```python
from build123d import *

# Parameters (mm, degrees)
SKETCH1_R           = 4
SKETCH1_R_2         = 1.7
SKETCH1_R_3         = 11
BOSS_EXTRUDE1_DEPTH = 3
FILLET1_R           = 10
SKETCH2_R           = 1.25
SKETCH2_R_2         = 1.255555556
CUT_EXTRUDE1_DEPTH  = 3


with BuildPart() as part:
    # Sketch1 → Boss-Extrude1 (new body)
    with BuildSketch(Plane(origin=(0, 0, 0), x_dir=(1, 0, 0), z_dir=(0, 1, 0))):
        Polygon((20, -64), (-20, -64), (-60, -7), (-60, 21.5), (-45.5, 50), (-31, 50), (-31, 19), (31, 19), (31, 50), (45.5, 50), (60, 21.5), (60, -7), align=None)
        with Locations((0, -10)):
            Circle(SKETCH1_R, mode=Mode.SUBTRACT)
        with Locations((-40, 0)):
            Circle(SKETCH1_R, mode=Mode.SUBTRACT)
        with Locations((40, 0)):
            Circle(SKETCH1_R, mode=Mode.SUBTRACT)
        with Locations((-15.5, -23.5)):
            Circle(SKETCH1_R_2, mode=Mode.SUBTRACT)
        with Locations((15.5, -23.5)):
            Circle(SKETCH1_R_2, mode=Mode.SUBTRACT)
        with Locations((15.5, -54.5)):
            Circle(SKETCH1_R_2, mode=Mode.SUBTRACT)
        with Locations((-15.5, -54.5)):
            Circle(SKETCH1_R_2, mode=Mode.SUBTRACT)
        with Locations((0, -39)):
            Circle(SKETCH1_R_3, mode=Mode.SUBTRACT)
    extrude(amount=BOSS_EXTRUDE1_DEPTH)

    # Fillet1
    fillet1_edges = [part.edges().sort_by_distance(p)[0] for p in [
        (45.5, 1.5, -50),
        (60, 1.5, -21.5),
        (60, 1.5, 7),
        (20, 1.5, 64),
        (-20, 1.5, 64),
        (-60, 1.5, 7),
        (-60, 1.5, -21.5),
        (-45.5, 1.5, -50),
    ]]
    fillet(fillet1_edges, radius=FILLET1_R)

    # Sketch2 → Cut-Extrude1 (cut)
    with BuildSketch(Plane(origin=(0, 3, 0), x_dir=(1, 0, 0), z_dir=(0, 1, 0))):
        with Locations((-32.400459523, -28.920654821)):
            Circle(SKETCH2_R)
        with Locations((32.400459523, -28.920654821)):
            Circle(SKETCH2_R)
        with Locations((0, 9)):
            Circle(SKETCH2_R)
        with Locations((-41, 36.792031786)):
            Circle(SKETCH2_R)
        with Locations((41, 36.792031786)):
            Circle(SKETCH2_R_2)
    extrude(amount=-CUT_EXTRUDE1_DEPTH, mode=Mode.SUBTRACT)


solid = part.part
```
Build history of the part. All positions in model axes, mm. A direction names the side the tool comes from. Round coordinates to 2 decimals unless told otherwise and drop trailing zeros. Write each loop counter-clockwise with the first axis right and the second up, starting at its lowest first coordinate (ties: lowest second). Pieces come first, ordered by that corner, then holes. Notation, with made-up numbers: (20.25, -7.75) - (41.25, -7.75) arc R21 cw to (41.25, 29.25) - close; hole circle Ø11 at (85, 56). An arc over 180 degrees is marked (long way). Answer as CSV lines item,"result".
Q1. Pull direction Z, two halves, no side cores. Call faces 3 (the cylindrical face through (-31.246, 1.521, 29.399)), 4 (the cylindrical face through (-19.354, 1.521, 62.903)), 5 (the cylindrical face through (17.07, 1.48, 55.15)), 6 (the flat face through (-35, 1, -50)): +Z half, -Z half, draft (parallel to the pull), parting line (faces both ways), or undercut.
Report:
face 3,"undercut"
face 4,"+Z half"
face 5,"undercut"
face 6,"-Z half"
Q2. Drill centre lines: probe 1 along Z at (x, y) = (0, 1.5); probe 2 along X at (y, z) = (2.45, 0); probe 3 along Z at (x, y) = (15.5, 1.25). Where is each one in solid material? Low to high. Write a range as [from, to].
Report:
probe 1,"z = [-19, -10.25], [-7.75, 6], [14, 28], [50, 64]"
probe 2,"x = [-60, -44], [-36, 36], [44, 60]"
probe 3,"z = [-19, 21.8], [25.2, 52.8], [56.2, 63.98]"
Q3. Tool access for faces 1 (the cylindrical face through (-43.2, 1.5, 2.4)), 2 (the flat face through (-31, 1, -35)): list every direction of +Z, -Z, +X, -X, +Y, -Y with a clear straight run to the whole face (end or side of a thin tool).
Report:
face 1,"+Y, -Y"
face 2,"-Z, +Y, -Y"
Q4. Cut at C-C (z = 54.5). Write the cut outline in (x, y).
Report:
outline,"(-26.67, 0) - (-17.2, 0) - (-17.2, 3) - (-26.67, 3) - close; (-13.8, 0) - (13.8, 0) - (13.8, 3) - (-13.8, 3) - close; (17.2, 0) - (26.67, 0) - (26.67, 3) - (17.2, 3) - close"
Q5. Cut at D-D (y = 0.45). State how many separate pieces and enclosed holes the cut face has, and give its area (3 significant figures).
Report:
separate pieces,"1"
enclosed holes,"13"
area,"8,450 mm^2"
Q6. Drop a flat-ended pin along its axis: pin 1 (0.9 mm diameter, centred on x = 12.5, y = 1.5, fed in from -Z). Give the stop position or say it passes through.
Report:
pin 1,"stops at z = -19"
Q7. Cut at B-B (z = 35.5). Write the cut outline in (x, y).
Report:
outline,"(-40, 0) - (-10.43, 0) - (-10.43, 3) - (-40, 3) - close; (10.43, 0) - (40, 0) - (40, 3) - (10.43, 3) - close"
Q8. Cut at A-A (x = 9). Write the cut outline in (y, z), and give its area (3 significant figures).
Report:
outline,"(0, -19) - (3, -19) - (3, 32.68) - (0, 32.68) - close; (0, 45.32) - (3, 45.32) - (3, 64) - (0, 64) - close"
area,"211 mm^2"
